Could you check a few things on this model? Use its own coordinates, in mm. A direction names the side the tool comes from. Give positions to 0.01 mm unless a question says otherwise; leave off trailing zeros. Loops run counter-clockwise (first coordinate to the right, second up) from the corner with the lowest first, then second, coordinate; pieces in that order, holes last. Notation, with made-up numbers: M -34.5,-5.75 L 13.5,-5.75 A5 ccw 13.5,-1.75 Z; hole C 73,48.5 d7. An arc over 180 degrees is marked long. Use a Markdown table: item, result. Add a question column.
1) If I drill on line 1 along X through (y, z) = (10.75, 47.75); line 2 along Y through (x, z) = (-133, 46); line 3 along Y through (x, z) = (-122, 46.75), over which ranges is the centre line in solid material (lowest first)? Write a range as [from, to].
2) Suppose I cut it at C-C on x = -117. List the corners of the cut face in (y, z) for me.
3) Suppose I cut it at A-A on y = 10.5. List the corners of the cut face in (x, z) for me, and give its area (3 significant figures).
4) Suppose I cut it at D-D on z = 47.25. Count the separate pieces of the cut face and the enclosed holes in it, and give its area (3 significant figures).
5) We'd pull the mould along X, two halves only. Please class faces 1 (the cylindrical face through (-110.987, 1.467, 48.737)), 2 (the flat face through (-121, 5, 42.824)), 3 (the flat face through (-106.047, 1, 48)), 4 (the flat face through (-136.047, 1, 48)): +X half, -X half, draft (parallel to the pull), parting line (faces both ways), or undercut.
6) Which directions (+Z, -Z, +X, -X, +Y, -Y) give clear straight access to the entire face, cutting with the end or side of a thin tool? Please do faces 5 (the flat face through (-108, 3, 48)), 6 (the flat face through (-121, 0, 48)), 7 (the flat face through (-128.547, 10, 48)).
7) Will these pins go through, and if not, where does the flat tip stop? pin 1 Ø1 at (y, z) = (8.5, 50) entering from -X; pin 2 Ø2.5 at (x, z) = (-109.8, 47.82) entering from +Y; pin 3 Ø6 at (x, z) = (-109, 45.5) entering from +Y.
8) Suppose I cut it at B-B on z = 45.75. List the corners of the cut face in (x, y) for me, and give its area (3 significant figures).
```python
from build123d import *

# Parameters (mm, degrees)
SKETCH1_W                       = 30
SKETCH1_H                       = 10
BOSS_EXTRUDE1_DEPTH             = 3
SKETCH2_W                       = 15
SKETCH2_H                       = 10
BOSS_EXTRUDE2_DEPTH             = 15
SKETCH3_R                       = 5
CUT_EXTRUDE1_DEPTH              = 138.595978597
F_3_0MM_DOWEL_HOLE1_D           = 3
F_3_0MM_DOWEL_HOLE1_CSINK_D     = 3.05
F_3_0MM_DOWEL_HOLE1_CSINK_ANGLE = 90


with BuildPart() as part:
    # Sketch1 → Boss-Extrude1 (new body)
    with BuildSketch(Plane(origin=(0, 0, 0), x_dir=(1, 0, 0), z_dir=(0, 1, 0))):
        with Locations((-121.046511628, -47.823920266)):
            Rectangle(SKETCH1_W, SKETCH1_H)
    extrude(amount=BOSS_EXTRUDE1_DEPTH)

    # Sketch2 → Boss-Extrude2 (add)
    with BuildSketch(Plane(origin=(0, 3, 0), x_dir=(1, 0, 0), z_dir=(0, 1, 0))):
        with Locations((-121.046511628, -47.823920266)):
            Rectangle(SKETCH2_W, SKETCH2_H)
    extrude(amount=BOSS_EXTRUDE2_DEPTH)

    # Sketch3 → Cut-Extrude1 (cut, through all)
    with BuildSketch(Plane.XY.offset(52.823920266)):
        with Locations((-121.046511628, 10.5)):
            Circle(SKETCH3_R)
    extrude(amount=-CUT_EXTRUDE1_DEPTH, mode=Mode.SUBTRACT)

    # Ø3.0mm Dowel Hole1 (through all)
    with Locations(Plane(origin=(0, 3, 0), x_dir=(1, 0, 0), z_dir=(0, 1, 0))):
        with Locations((-132.296511628, -47.823920266)):
            f_3_0mm_dowel_hole1 = CounterSinkHole(F_3_0MM_DOWEL_HOLE1_D / 2, F_3_0MM_DOWEL_HOLE1_CSINK_D / 2, counter_sink_angle=F_3_0MM_DOWEL_HOLE1_CSINK_ANGLE)

    # Mirror1: Ø3.0mm Dowel Hole1 across plane
    add(f_3_0mm_dowel_hole1.mirror(Plane(origin=(-121.046511628, 0, 0), x_dir=(0, 0, 1), z_dir=(1, 0, 0))), mode=Mode.SUBTRACT)


solid = part.part
```
Answer block:
| question | item | result |
|---|---|---|
| 1 | line 1 | x = [-128.55, -126.04], [-116.05, -113.55] |
| 1 | line 2 | y = [0, 3] |
| 1 | line 3 | y = [0, 5.59], [15.41, 18] |
| 2 | outline | M 0,42.82 L 7.56,42.82 L 7.56,52.82 L 0,52.82 Z; M 13.44,42.82 L 18,42.82 L 18,52.82 L 13.44,52.82 Z |
| 3 | outline | M -128.55,42.82 L -126.05,42.82 L -126.05,52.82 L -128.55,52.82 Z; M -116.05,42.82 L -113.55,42.82 L -113.55,52.82 L -116.05,52.82 Z |
| 3 | area | 50.0 mm^2 |
| 4 | separate pieces | 3 |
| 4 | enclosed holes | 1 |
| 4 | area | 220 mm^2 |
| 5 | face 1 | undercut |
| 5 | face 2 | draft |
| 5 | face 3 | +X half |
| 5 | face 4 | -X half |
| 6 | face 5 | +Z, -Z, +X, +Y |
| 6 | face 6 | +Z, -Z, +X, -X, -Y |
| 6 | face 7 | +Z, -Z, -X, +Y |
| 7 | pin 1 | stops at x = -128.55 |
| 7 | pin 2 | passes through |
| 7 | pin 3 | stops at y = 3 |
| 8 | outline | M -136.05,0 L -106.05,0 L -106.05,3 L -113.55,3 L -113.55,18 L -128.55,18 L -128.55,3 L -136.05,3 Z; hole C -121.05,10.5 d10 |
| 8 | area | 236 mm^2 |
